from build123d import *

# Parameters (mm, degrees)
ESQUISSE1_W             = 2.5
ESQUISSE1_H             = 10
BOSS_EXTRU_1_DEPTH      = 7
BOSS_EXTRU_2_DEPTH      = 3
BOSS_EXTRU_2_DEPTH_BACK = 10
ENL_V_MAT_EXTRU_1_REACH = 44.024
ESQUISSE4_4_W           = 7
ESQUISSE4_4_H           = 9.399494937
ENL_V_MAT_EXTRU_4_DEPTH = 3
ENL_V_START             = -13
ESQUISSE4_W             = 7
ESQUISSE4_H             = 9.399494937
ENL_V_MAT_EXTRU_2_DEPTH = 3
CHANFREIN1_SIZE         = 3
CONG_1_R                = 1
ESQUISSE5_R             = 4.8
ENL_V_MAT_EXTRU_5_DEPTH = 1
ESQUISSE6_R             = 2.5
ESQUISSE6_R_2           = 2
ENL_V_MAT_EXTRU_6_DEPTH = 42.047043387
CHANFREIN2_SIZE         = 1
SKETCH_1_W              = 7
SKETCH_1_H              = 5
CUT_EXTRUDE_1_DEPTH     = 1
SKETCH_2_W              = 7
SKETCH_2_H              = 5
CUT_EXTRUDE_2_DEPTH     = 1
EXTRUDE_1_DEPTH         = 3
FILLET_1_R              = 3
FILLET_2_R              = 1
FILLET_3_R              = 2
CUT_EXTRUDE_START       = -30
SKETCH_5_R              = 3
CUT_EXTRUDE_3_DEPTH     = 30


# Some blends are built 0.0001 mm under size
with BuildPart() as part:
    # Esquisse1 → Boss.-Extru.1 (new body)
    with BuildSketch(Plane.XY):
        Polygon((-8, 6), (-16, 6), (-16, 1), (-16, -9), (-16, -24), (-21, -24), (-7.5, -34), (0, -34), (0, 0), (-2, 0), align=None)
        Polygon((2, 0), (0, 0), (0, -34), (7.5, -34), (21, -24), (16, -24), (16, -9), (16, 1), (16, 6), (8, 6), align=None)
        with Locations((17.25, -4)):
            Rectangle(ESQUISSE1_W, ESQUISSE1_H)
        with Locations((-17.25, -4)):
            Rectangle(ESQUISSE1_W, ESQUISSE1_H)
    extrude(amount=BOSS_EXTRU_1_DEPTH)

    # Esquisse2 → Boss.-Extru.2 (add, two sides: drawn at the far end of the back side and taken through both)
    with BuildSketch(Plane.XY.offset(7).offset(-BOSS_EXTRU_2_DEPTH_BACK)):
        Polygon((16, -14), (-16, -14), (-16, -24), (-21, -24), (-7.5, -34), (7.5, -34), (21, -24), (16, -24), align=None)
    extrude(amount=BOSS_EXTRU_2_DEPTH + BOSS_EXTRU_2_DEPTH_BACK)

    # Esquisse3 → Enlèv. mat.-Extru.1 (cut, up to next)
    with BuildSketch(Plane(origin=(0, 0, -3), x_dir=(-1, 0, 0), z_dir=(0, 0, -1)), mode=Mode.PRIVATE) as enl_v_mat_extru_1_sk1:
        Polygon((-11, -0.899494937), (-3.5, -8.399494937), (-3.5, -23.399494937), (-11, -15.899494937), align=None)
    enl_v_mat_extru_1_tool1 = extrude(enl_v_mat_extru_1_sk1.sketch, amount=-ENL_V_MAT_EXTRU_1_REACH, mode=Mode.PRIVATE) & part.part
    # Esquisse3 → Enlèv. mat.-Extru.1 (cut, up to next)
    with BuildSketch(Plane(origin=(0, 0, -3), x_dir=(-1, 0, 0), z_dir=(0, 0, -1)), mode=Mode.PRIVATE) as enl_v_mat_extru_1_sk2:
        Polygon((11, -15.899494937), (11, -0.899494937), (3.5, -8.399494937), (3.5, -23.399494937), align=None)
    enl_v_mat_extru_1_tool2 = extrude(enl_v_mat_extru_1_sk2.sketch, amount=-ENL_V_MAT_EXTRU_1_REACH, mode=Mode.PRIVATE) & part.part
    add(enl_v_mat_extru_1_tool1.solids().sort_by_distance((7.25, -12.149495, -3))[0], mode=Mode.SUBTRACT)
    add(enl_v_mat_extru_1_tool2.solids().sort_by_distance((-7.25, -12.149495, -3))[0], mode=Mode.SUBTRACT)

    # Esquisse4<4> → Enlèv. mat.-Extru.4 (cut)
    with BuildSketch(Plane(origin=(0, 0, -3), x_dir=(-1, 0, 0), z_dir=(0, 0, -1))):
        with Locations((0, -18.699747469)):
            Rectangle(ESQUISSE4_4_W, ESQUISSE4_4_H)
    extrude(amount=-ENL_V_MAT_EXTRU_4_DEPTH, mode=Mode.SUBTRACT)

    # Esquisse4 → Enlèv. mat.-Extru.2 (cut)
    with BuildSketch(Plane(origin=(0, 0, -3), x_dir=(-1, 0, 0), z_dir=(0, 0, -1)).offset(ENL_V_START)):
        with Locations((0, -18.699747469)):
            Rectangle(ESQUISSE4_W, ESQUISSE4_H)
    extrude(amount=ENL_V_MAT_EXTRU_2_DEPTH, mode=Mode.SUBTRACT)

    # Chanfrein1
    chanfrein1_edges = [part.edges().sort_by_distance(p)[0] for p in [
        (-13.5, -14, 0),
        (-13.5, -14, 7),
        (13.5, -14, 0),
        (13.5, -14, 7),
    ]]
    chamfer(chanfrein1_edges, length=CHANFREIN1_SIZE - 0.0001)  # a hair under: the kernel refuses the full size

    # Congé1
    cong_1_edges = [part.edges().sort_by_distance(p)[0] for p in [
        (11, -15.899494937, 3.5),
        (11, -0.899494937, 3.5),
        (-11, -0.899494937, 3.5),
        (-11, -15.899494937, 3.5),
        (-21, -24, 3.5),
        (21, -24, 3.5),
    ]]
    fillet(cong_1_edges, radius=CONG_1_R)

    # Esquisse5 → Enlèv. mat.-Extru.5 (cut)
    with BuildSketch(Plane.XZ.offset(34)):
        with Locations(Location((0, 3.5, 0), (0, 0, 270))):
            Circle(ESQUISSE5_R)
    extrude(amount=-ENL_V_MAT_EXTRU_5_DEPTH, mode=Mode.SUBTRACT)

    # Esquisse6 → Enlèv. mat.-Extru.6 (cut, through all)
    with BuildSketch(Plane.XY.offset(10)):
        with Locations((-10, -24)):
            Circle(ESQUISSE6_R)
        with Locations((0, -28.5)):
            Circle(ESQUISSE6_R_2)
        with Locations(Location((10, -24, 0), (0, 0, 180))):
            Circle(ESQUISSE6_R)
    extrude(amount=-ENL_V_MAT_EXTRU_6_DEPTH, mode=Mode.SUBTRACT)

    # Chanfrein2
    chanfrein2_edges = [part.edges().sort_by_distance(p)[0] for p in [
        (0, -34, -3),
        (0, -34, 10),
    ]]
    chamfer(chanfrein2_edges, length=CHANFREIN2_SIZE)

    # Эскиз1 → Вырез-Вытянуть1 (cut)
    with BuildSketch(Plane(origin=(16, 0, 0), x_dir=(0, 0, -1), z_dir=(1, 0, 0))):
        with Locations((-3.5, 3.5)):
            Rectangle(SKETCH_1_W, SKETCH_1_H)
        Polygon((-10, -24), (3, -24), (3, -14), (0, -11), (0, -9), (-7, -9), (-7, -11), (-10, -14), align=None)
    extrude(amount=-CUT_EXTRUDE_1_DEPTH, mode=Mode.SUBTRACT)

    # Эскиз2 → Вырез-Вытянуть2 (cut)
    with BuildSketch(Plane.ZY.offset(16)):
        with Locations((3.5, 3.5)):
            Rectangle(SKETCH_2_W, SKETCH_2_H)
        Polygon((10, -24), (10, -14), (7, -11), (7, -9), (0, -9), (0, -11), (-3, -14), (-3, -24), align=None)
    extrude(amount=-CUT_EXTRUDE_2_DEPTH, mode=Mode.SUBTRACT)

    # Эскиз4 → Бобышка-Вытянуть1 (add)
    with BuildSketch(Plane(origin=(0, 0, 0), x_dir=(-1, 0, 0), z_dir=(0, 0, -1))):
        with BuildLine():
            Line((15, -14), (15, -11))
            Line((15, -11), (15, -9))
            Line((15, -9), (15, 6))
            Line((15, 6), (8, 6))
            Line((8, 6), (2, 0))
            Line((2, 0), (-2, 0))
            Line((-2, 0), (-8, 6))
            Line((-8, 6), (-15, 6))
            Line((-15, 6), (-15, -9))
            Line((-15, -9), (-15, -11))
            Line((-15, -11), (-15, -14))
            Line((-15, -14), (-11, -14))
            Line((-11, -14), (-11, -11))
            Line((-11, -11), (-11, -3.313708499))
            ThreePointArc((-11, -3.313708499), (-10.382683432, -2.389828966), (-9.292893219, -2.606601718))
            Line((-9.292893219, -2.606601718), (-3.5, -8.399494937))
            Line((-3.5, -8.399494937), (-3.5, -23.399494937))
            Line((-3.5, -23.399494937), (3.5, -23.399494937))
            Line((3.5, -23.399494937), (3.5, -8.399494937))
            Line((3.5, -8.399494937), (9.292893219, -2.606601718))
            ThreePointArc((9.292893219, -2.606601718), (10.382683432, -2.389828966), (11, -3.313708499))
            Line((11, -3.313708499), (11, -11))
            Line((11, -11), (11, -14))
            Line((11, -14), (15, -14))
        make_face()
    extrude(amount=EXTRUDE_1_DEPTH)

    # Скругление1
    fillet_1_edges = [part.edges().sort_by_distance(p)[0] for p in [
        (-7.5, -34, 3.5),
        (7.5, -34, 3.5),
    ]]
    fillet(fillet_1_edges, radius=FILLET_1_R)

    # Скругление2
    fillet_2_edges = [part.edges().sort_by_distance(p)[0] for p in [
        (15, -24, 3.5),
        (-15, -24, 3.5),
    ]]
    fillet(fillet_2_edges, radius=FILLET_2_R)

    # Скругление3
    fillet_3_edges = [part.edges().sort_by_distance(p)[0] for p in [
        (3.5, -8.399494937, 2),
        (-3.5, -8.399494937, 2),
    ]]
    fillet(fillet_3_edges, radius=FILLET_3_R)

    # Скругление4
    # a fillet whose section is not a circle: 2 mm, written as the material it adds along each edge
    with BuildSketch(Plane(origin=(-3.5, -23.399494937, 7), x_dir=(0, 1, 0), z_dir=(0, 0, -1)), Plane(origin=(3.5, -23.399494937, -3), x_dir=(0, 1, 0), z_dir=(0, 0, 1))) as fillet_4_piece_1:
        with BuildLine():
            Bezier((4.828427125, 0), (0, 0), (3.414213562, -3.414213562), weights=[1, 1, 1])
            Line((3.414213562, -3.414213562), (0, 0))
            Line((0, 0), (4.828427125, 0))
        make_face()
    extrude(amount=10)

    # Эскиз5 → Вырез-Вытянуть3 (cut)
    with BuildSketch(Plane.ZY.offset(15).offset(CUT_EXTRUDE_START)):
        with Locations((-3.39031082, -5.412141647)):
            Circle(SKETCH_5_R)
    extrude(amount=CUT_EXTRUDE_3_DEPTH, mode=Mode.SUBTRACT)


solid = part.part
Model file for the job. Use its own axes, mm. A direction names the side the tool comes from. Coordinates: 2 decimals unless noted, no trailing zeros. Order: outer loops, then holes, each group sorted by start corner. A loop starts at its lowest first (then second) coordinate and runs counter-clockwise, first axis right, second up. Notation, with made-up numbers: (44, -9) -> (91, -9) arc R26 cw to (91, 5) -> close; hole circle Ø8 at (-9, 24). An arc over 180 degrees is marked (long way). Return JSON: item names as keys, results as strings. Group by question number.
Item 1: Saw through at C-C on x = 10. Write the cut outline in (y, z), then the cut area to 3 significant figures.
Item 2: Saw through at B-B on y = -15. Write the cut outline in (x, z), then the cut area to 3 significant figures.
Item 3: Wall check: line 1 along Y through (x, z) = (0, 1); line 2 along X through (y, z) = (-16.5, 3.5); line 3 along X through (y, z) = (-3, 6.5). Give the ranges that are in metal, low to high. Write a range as [from, to].
Item 4: Pull direction Y, two halves, no side cores. Call faces 4 (the flat face through (-5, 3, 2)), 5 (the cylindrical face through (-7.463, -33.845, 3.585)), 6 (the cylindrical face through (15.285, -23.699, 3.409)), 7 (the flat face through (-17, -9, 4)): pulls with the +Y half, pulls with the -Y half, needs draft (parallel to the pull), parting line crosses it, or undercut.
Item 5: Saw through at D-D on z = 4. State how many separate pieces and enclosed holes the cut face has, then the cut area to 3 significant figures.
Item 6: Saw through at A-A on y = 2. Write the cut outline in (x, z).
Item 7: Flat gauge pins, fed straight in: P1, Ø3, axis at y = -1.5, z = 5.5, coming from the -X side; P2, Ø5, axis at x = -6, y = -1, coming from the +Z side; P3, Ø4, axis at x = -17.5, z = 3.5, coming from the -Y side. Where does each tip first touch, or does it go through?
Item 8: Tool access for faces 1 (the flat face through (-11, -11, 3)), 2 (the flat face through (-17, -24, 3)), 3 (the flat face through (0, 0, 2)): list every direction of +Z, -Z, +X, -X, +Y, -Y with a clear straight run to the whole face (end or side of a thin tool).
Values found:
{
 "1": {"outline": "(-32.15, -3) -> (-26.5, -3) -> (-26.5, 10) -> (-32.15, 10) -> close; (-21.5, -3) -> (-16.9, -3) -> (-16.9, 10) -> (-21.5, 10) -> close; (-2.31, -3) -> (6, -3) -> (6, 7) -> (-2.31, 7) -> close", "area": "216 mm2"},
 "2": {"outline": "(-15, -3) -> (-11, -3) -> (-11, 10) -> (-15, 10) -> close; (-3.5, -3) -> (3.5, -3) -> (3.5, 7) -> (-3.5, 7) -> close; (11, -3) -> (15, -3) -> (15, 10) -> (11, 10) -> close", "area": "174 mm2"},
 "3": {"line 1": "y = [-33, -30.5], [-26.5, 0]", "line 2": "x = [-15, -10.4], [-3.5, 3.5], [10.4, 15]", "line 3": "x = [-18.5, -10.95], [-8.9, 8.9], [10.95, 18.5]"},
 "4": {"face 4": "pulls with the +Y half", "face 5": "pulls with the -Y half", "face 6": "undercut", "face 7": "undercut"},
 "5": {"separate pieces": "1", "enclosed holes": "5", "area": "913 mm2"},
 "6": {"outline": "(-15, -3) -> (-4, -3) -> (-4, 7) -> (-15, 7) -> close; (4, -3) -> (15, -3) -> (15, 7) -> (4, 7) -> close"},
 "7": {"P1": "stops at x = -18.5", "P2": "stops at z = 7", "P3": "stops at y = -28.07"},
 "8": {"face 1": "+Z, -Z", "face 2": "+Z, -Z, -X", "face 3": "+Z, -Z, +Y"}
}
